The model under review builds one solid part; all positions refer to its coordinate system, in mm. Give positions to 0.01 mm unless a question says otherwise; leave off trailing zeros. Write each loop counter-clockwise with the first axis right and the second up, starting at its lowest first coordinate (ties: lowest second). Pieces come first, ordered by that corner, then holes. Notation, with made-up numbers: M -35,22 L 21,22 A34 cw 21,60 Z; hole C -32,55 d3. An arc over 180 degrees is marked long. Write item = value, one per line. Start each with the question number.
```python
from build123d import *

# Parameters (mm, degrees)
SKETCH1_R           = 68.369999998
SKETCH1_R_2         = 23.401
BOSS_EXTRUDE1_DEPTH = 1
SKETCH2_R           = 1.5
CUT_EXTRUDE1_DEPTH  = 10
SKETCH6_R           = 5
CUT_EXTRUDE2_DEPTH  = 10


with BuildPart() as part:
    # Sketch1 → Boss-Extrude1 (new body)
    with BuildSketch(Plane(origin=(0, 0, 0), x_dir=(-1, 0, 0), z_dir=(0, 1, 0))):
        with Locations(Location((-73.249601195, 33.216650322, 0), (0, 0, 90))):
            Circle(SKETCH1_R)
        with Locations(Location((-73.249601195, 33.216650322, 0), (0, 0, 90))):
            Circle(SKETCH1_R_2, mode=Mode.SUBTRACT)
    extrude(amount=BOSS_EXTRUDE1_DEPTH)

    # Sketch2 → Cut-Extrude1 (cut)
    with BuildSketch(Plane.XZ.offset(-1)):
        with Locations(Location((18.303061139, 35.641054554, 0), (0, 0, 90))):
            Circle(SKETCH2_R)
        with Locations(Location((102.822466876, 79.589547745, 0), (0, 0, 90))):
            Circle(SKETCH2_R)
        with Locations(Location((98.623275569, -15.580651332, 0), (0, 0, 90))):
            Circle(SKETCH2_R)
    extrude(amount=CUT_EXTRUDE1_DEPTH, mode=Mode.SUBTRACT)

    # Sketch6 → Cut-Extrude2 (cut)
    with BuildSketch(Plane(origin=(47.341973048, -2, 109.358916756), x_dir=(0.09761667308977556, 0, 0.995224087899245), z_dir=(0, -1, 0))):
        with Locations(Location((-105.702188225, -2.042468777, 0), (0, 0, 5.601944352))):
            Circle(SKETCH6_R)
        with Locations(Location((-44.324158759, 1.255349618, 0), (0, 0, 5.601944352))):
            Circle(SKETCH6_R)
    extrude(amount=-CUT_EXTRUDE2_DEPTH, mode=Mode.SUBTRACT)


solid = part.part
```
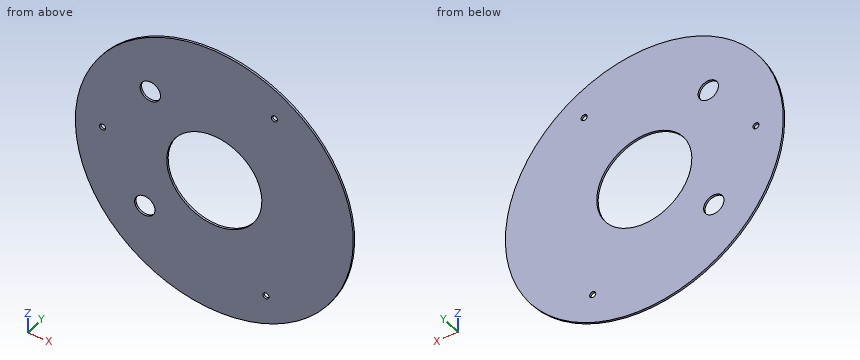
Item 1: We need section A-A, the plane x = 86. Write out the cut boundary in (y, z), and give its area (3 significant figures).
Item 2: Clearance check with a flat-ended pin moving along its axis: P1, Ø8, axis at x = 39.06, z = 3.96, coming from the -Y side. State where the tip first meets the part, or that it passes through.
Item 3: We need section D-D, the plane z = 91. Write out the cut boundary in (x, y).
Item 4: We need section C-C, the plane y = 0.4. Write out the cut boundary in (x, z), and give its area (3 significant figures).
Item 5: To check wall thickness, follow probe 1 along Z at (x, y) = (38, 0.6); probe 2 along X at (y, z) = (0.25, 36); probe 3 along X at (y, z) = (0.35, 53.5). State the ranges of each line that lie inside material, in increasing order. Write a range as [from, to].
Item 6: We need section B-B, the plane z = 21.5. Write out the cut boundary in (x, y), and give its area (3 significant figures).
Worked out:
q1.outline = M 0,-33.95 L 1,-33.95 L 1,13.59 L 0,13.59 Z; M 0,52.84 L 1,52.84 L 1,100.39 L 0,100.39 Z
q1.area = 95.1 mm²
q2.P1 = through
q3.outline = M 36.7,0 L 109.79,0 L 109.79,1 L 36.7,1 Z
q4.outline = C 73.25,33.22 d136.74; hole C 18.3,35.64 d3; hole C 39.06,3.96 d10; hole C 41.77,65.37 d10; hole C 73.25,33.22 d46.8; hole C 98.62,-15.58 d3; hole C 102.82,79.59 d3
q4.area = 12,800 mm²
q5.probe_1 = [-25.37, -0.92], [8.85, 62.08], [68.66, 91.8]
q5.probe_2 = [4.94, 16.85], [19.76, 50.01], [96.48, 141.56]
q5.probe_3 = [7.96, 61.58], [84.92, 138.54]
q6.outline = M 5.89,0 L 52.99,0 L 52.99,1 L 5.89,1 Z; M 93.51,0 L 140.61,0 L 140.61,1 L 93.51,1 Z
q6.area = 94.2 mm²
